from build123d import *

# Parameters (mm, degrees)
F0_W     = 63.5
F0_H     = 38.1
F1_DEPTH = 25.4
F2_W     = 6.35
F2_H     = 38.1
F3_DEPTH = 19.05
F5_W     = 6.35
F5_H     = 19.05
F6_DEPTH = 38.101
F7_R     = 12.701006
F8_DEPTH = 25.401


with BuildPart() as f1:
    # F0 (on Top) → F1 (new body)
    with BuildSketch(Plane.XY):
        with Locations((-4.211051, 0.752282)):
            Rectangle(F0_W, F0_H)
    extrude(amount=F1_DEPTH)

    # F2 (on face) → F3 (cut)
    with BuildSketch(Plane.XY.offset(25.4)):
        with Locations((-32.786051, 0.752282)):
            Rectangle(F2_W, F2_H)
    extrude(amount=-F3_DEPTH, mode=Mode.SUBTRACT)

    # F5 (on face) → F6 (cut, through all)
    with BuildSketch(Plane(origin=(0, 19.802282, 0), x_dir=(-1, 0, 0), z_dir=(0, 1, 0))):
        with Locations((-24.363949, 15.875)):
            Rectangle(F5_W, F5_H)
    extrude(amount=-F6_DEPTH, mode=Mode.SUBTRACT)

    # F7 (on face) → F8 (cut, through all)
    with BuildSketch(Plane.XY.offset(25.4)):
        with Locations((-2.940286, 19.802282)):
            Circle(F7_R)
    extrude(amount=-F8_DEPTH, mode=Mode.SUBTRACT)


solid = f1.part
Verification items for the finished model (mm, model axes). A direction names the side the tool comes from. Coordinates: 2 decimals unless noted, no trailing zeros. Order: outer loops, then holes, each group sorted by start corner. A loop starts at its lowest first (then second) coordinate and runs counter-clockwise, first axis right, second up.
1. Release check for a two-part mould opening along X. For faces 4 (the face through (27.539, 0, 3)), 5 (the face through (17, 19.802, 13)), 6 (the face through (-3.22, 7.104, 12.878)) record: +X half, -X half, draft (parallel to the pull), parting line (faces both ways), or undercut.
Results found:
face 4: +X half
face 5: draft
face 6: undercut
2. Set-up check for faces 1 (the face through (-33, 1, 6.35)), 2 (the face through (24, 1, 6.35)), 3 (the face through (-35.961, 0, 3)): record each of +Z, -Z, +X, -X, +Y, -Y from which the full face is reachable in a straight line by a thin tool's end or side.
Results found:
face 1: +Z, -X, +Y, -Y
face 2: +Z, +X, +Y, -Y
face 3: +Z, -Z, -X, +Y, -Y
3. Scan lines: line 1 (X direction, y = 15.5, z = 8.75); line 2 (X direction, y = -13, z = 17.25); line 3 (Z direction, x = 22, y = 10.5). Record each from-to range of solid material in increasing order.
Results found:
line 1: x = -29.61 to -14.89, 9.01 to 21.19
line 2: x = -29.61 to 21.19
line 3: z = 0 to 6.35
4. Sectioned sample at A-A, the plane y = -14. Record the cut outline in (x, z), and give its area (3 significant figures).
Results found:
outline: (-35.96, 0) - (27.54, 0) - (27.54, 6.35) - (21.19, 6.35) - (21.19, 25.4) - (-29.61, 25.4) - (-29.61, 6.35) - (-35.96, 6.35) - close
area: 1,370 mm2
5. Sectioned sample at C-C, the plane y = 8. Record the cut outline in (x, z).
Results found:
outline: (-35.96, 0) - (-7.63, 0) - (-7.63, 25.4) - (-29.61, 25.4) - (-29.61, 6.35) - (-35.96, 6.35) - close; (1.75, 0) - (27.54, 0) - (27.54, 6.35) - (21.19, 6.35) - (21.19, 25.4) - (1.75, 25.4) - close
6. Sectioned sample at B-B, the plane z = 22. Record the cut outline in (x, y).
Results found:
outline: (-29.61, -18.3) - (21.19, -18.3) - (21.19, 19.8) - (9.76, 19.8) arc R12.7 cw to (-15.64, 19.8) - (-29.61, 19.8) - close
7. Sectioned sample at D-D, the plane x = 3. Record the cut outline in (y, z), and give its area (3 significant figures).
Results found:
outline: (-18.3, 0) - (8.58, 0) - (8.58, 25.4) - (-18.3, 25.4) - close
area: 683 mm2
8. Go/stop test with flat-tipped pins: pin 1 Ø7 at (x, y) = (-31.5, 5) entering from +Z; pin 2 Ø6 at (y, z) = (-12, 19) entering from -X; pin 3 Ø5 at (x, y) = (24, 0.5) entering from +Z. Record where each tip stops, or that it passes through.
Results found:
pin 1: stops at z = 25.4
pin 2: stops at x = -29.61
pin 3: stops at z = 6.35
